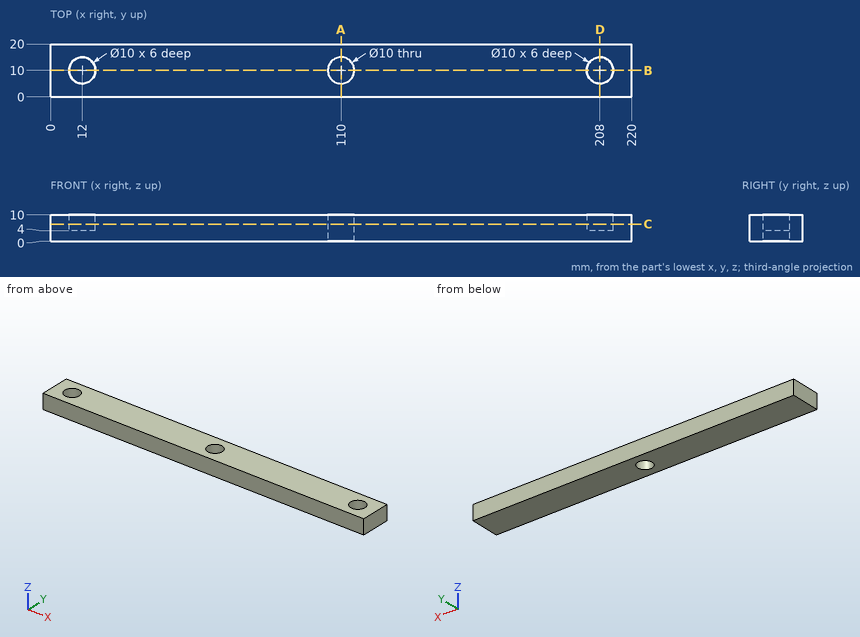
Here's the drawing with two shaded views (mm, measured from the low corner). I have some questions. Give positions to 0.01 mm unless a question says otherwise; leave off trailing zeros. Order: outer loops, then holes, each group sorted by start corner. A loop starts at its lowest first (then second) coordinate and runs counter-clockwise, first axis right, second up. Notation, with made-up numbers: (-5, 65) - (29, 65) arc R25 ccw to (29, 88) - close; hole circle Ø8 at (-24.75, -0.5). An arc over 180 degrees is marked (long way). Use a Markdown table: item, result. Add a question column.
Q1. If we section it at C-C on z = 6.5: Write out the boundary of the cut face in (x, y).
Q2. If we section it at B-B on y = 10: Write out the boundary of the cut face in (x, z).
Q3. If we section it at A-A on x = 110: Write out the boundary of the cut face in (y, z), plus the area to 3 significant figures.
Q4. I'm going to push flat-ended pins straight in: pin 1 (3 mm diameter, centred on x = 9.5, y = 12, fed in from +Z); pin 2 (6 mm diameter, centred on x = 110, y = 10, fed in from +Z). Where does each tip first touch, or does it pass through?
Q5. Please list where these lines run through material, in increasing order: line 1 along Y through (x, z) = (12, 7.75); line 2 along X through (y, z) = (6.25, 9.5); line 3 along X through (y, z) = (8.5, 7.75).
Q6. If we section it at D-D on x = 208: Write out the boundary of the cut face in (y, z), plus the area to 3 significant figures.
Answers follow:
| question | item | result |
|---|---|---|
| 1 | outline | (0, 0) - (220, 0) - (220, 20) - (0, 20) - close; hole circle Ø10 at (12, 10); hole circle Ø10 at (110, 10); hole circle Ø10 at (208, 10) |
| 2 | outline | (0, 0) - (105, 0) - (105, 10) - (17, 10) - (17, 4) - (7, 4) - (7, 10) - (0, 10) - close; (115, 0) - (220, 0) - (220, 10) - (213, 10) - (213, 4) - (203, 4) - (203, 10) - (115, 10) - close |
| 3 | outline | (0, 0) - (5, 0) - (5, 10) - (0, 10) - close; (15, 0) - (20, 0) - (20, 10) - (15, 10) - close |
| 3 | area | 100 mm^2 |
| 4 | pin 1 | stops at z = 4 |
| 4 | pin 2 | passes through |
| 5 | line 1 | y = 0 to 5, 15 to 20 |
| 5 | line 2 | x = 0 to 8.69, 15.31 to 106.69, 113.31 to 204.69, 211.31 to 220 |
| 5 | line 3 | x = 0 to 7.23, 16.77 to 105.23, 114.77 to 203.23, 212.77 to 220 |
| 6 | outline | (0, 0) - (20, 0) - (20, 10) - (15, 10) - (15, 4) - (5, 4) - (5, 10) - (0, 10) - close |
| 6 | area | 140 mm^2 |
